Answer from the drawing. Dimensions are ordinates in mm from the lowest x, y and z of the part. A direction names the side the tool comes from. Coordinates: 2 decimals unless noted, no trailing zeros. Write each loop counter-clockwise with the first axis right and the second up, starting at its lowest first coordinate (ties: lowest second). Pieces come first, ordered by that corner, then holes. Notation, with made-up numbers: (14, 84.5) -> (62, 84.5) arc R18 ccw to (62, 94.5) -> close; hole circle Ø9 at (32.5, -32). An arc over 180 degrees is marked (long way). One line per item, written item: value. Start each with the question number.
1. For a pull along X with two mould halves and no side action, classify the marked faces 1, 2 and 3 as pulls with the +X half, pulls with the -X half, needs draft (parallel to the pull), parting line crosses it, or undercut.
2. Find section B-B, the plane y = 35.5. Write down the section's boundary in (x, z).
3. Find section D-D, the plane y = 20.5. Write down the section's boundary in (x, z), and give its area (3 significant figures).
4. Given P1, Ø2, axis at y = 10, z = 10, coming from the -X side; P2, Ø3, axis at x = 8.5, z = 4, coming from the +Y side; P3, Ø1.8, axis at x = 4, z = 6, coming from the -Y side, each flat-ended and moving along its own axis, determine where each tip first touches the part or whether it passes through.
5. Find section C-C, the plane x = 9. Write down the section's boundary in (y, z), and give its area (3 significant figures).
6. Consider line 1 along X through (y, z) = (11.5, 11.75); line 2 along Y through (x, z) = (24, 11.5); line 3 along Z through (x, y) = (4, 25.5). Determine where each line is inside the solid, lowest interval first.
7. Find section A-A, the plane z = 1.5. Write down the section's boundary in (x, y) (1 decimal).
8. For the marked faces 4, 5, 6 and 7, determine the directions among +Z, -Z, +X, -X, +Y, -Y from which every point of the face is accessible in a straight line to the end or side of a thin tool.
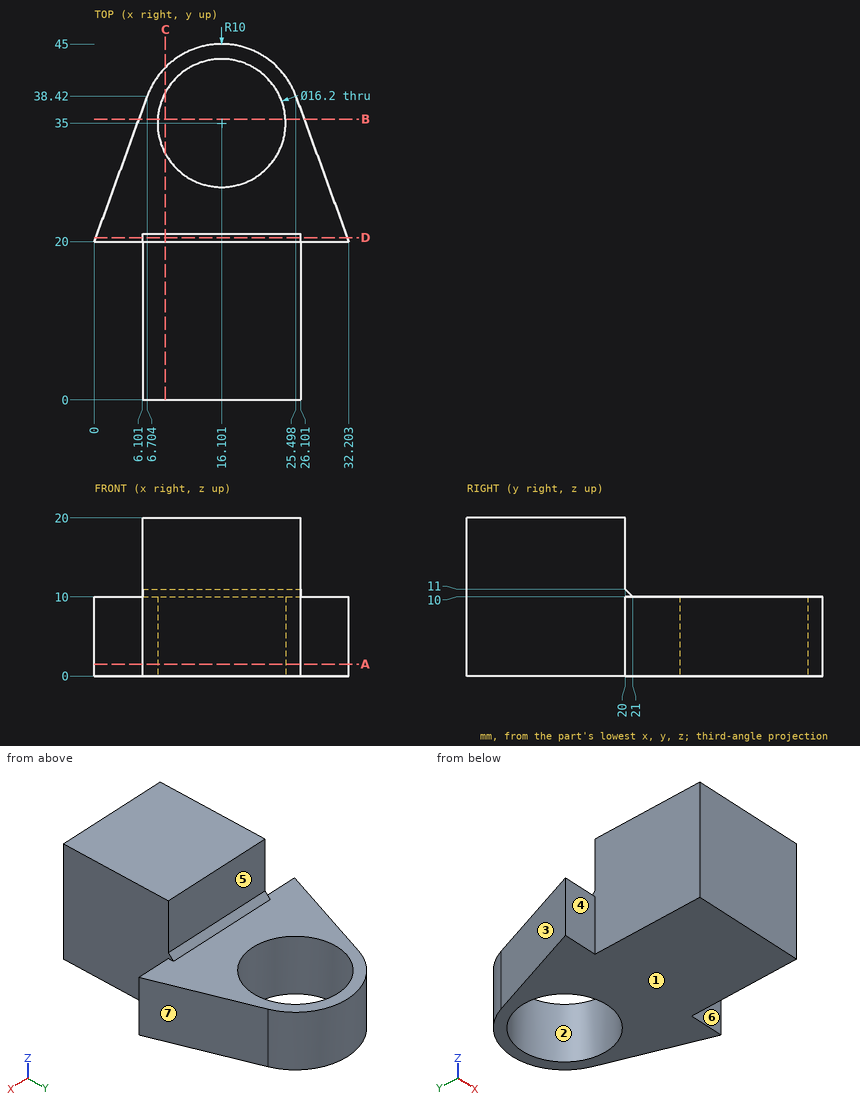
Answer block:
1. face 1: needs draft
1. face 2: undercut
1. face 3: pulls with the -X half
2. outline: (5.64, 0) -> (8.02, 0) -> (8.02, 10) -> (5.64, 10) -> close; (24.19, 0) -> (26.56, 0) -> (26.56, 10) -> (24.19, 10) -> close
3. outline: (0.18, 0) -> (32.02, 0) -> (32.02, 10) -> (26.1, 10) -> (26.1, 10.5) -> (6.1, 10.5) -> (6.1, 10) -> (0.18, 10) -> close
3. area: 328 mm2
4. P1: stops at x = 6.1
4. P2: stops at y = 42.92
4. P3: stops at y = 20
5. outline: (0, 0) -> (31.1, 0) -> (31.1, 10) -> (21, 10) -> (20, 11) -> (20, 20) -> (0, 20) -> close; (38.9, 0) -> (42.04, 0) -> (42.04, 10) -> (38.9, 10) -> close
5. area: 543 mm2
6. line 1: x = 6.1 to 26.1
6. line 2: y = 0 to 20
6. line 3: z = 0 to 10
7. outline: (0, 20) -> (6.1, 20) -> (6.1, 0) -> (26.1, 0) -> (26.1, 20) -> (32.2, 20) -> (25.5, 38.4) arc R10 ccw to (6.7, 38.4) -> close; hole circle Ø16.2 at (16.1, 35)
8. face 4: +Z, -Z, -X, -Y
8. face 5: +Z, +X, -X, +Y
8. face 6: +Z, -Z, +X, -Y
8. face 7: +Z, -Z, +X, +Y
